Part print with two shaded views. Sizes in mm from the minimum x, y, z corner. A direction names the side the tool comes from. Round coordinates to 2 decimals unless told otherwise and drop trailing zeros. Order: outer loops, then holes, each group sorted by start corner. A loop starts at its lowest first (then second) coordinate and runs counter-clockwise, first axis right, second up. Notation, with made-up numbers: M 37.25,-13 L 77.25,-13 A8 cw 77.25,-7 Z; hole C 89,89.5 d9. An arc over 180 degrees is marked long. Answer as a JSON object with one key per item and string values.
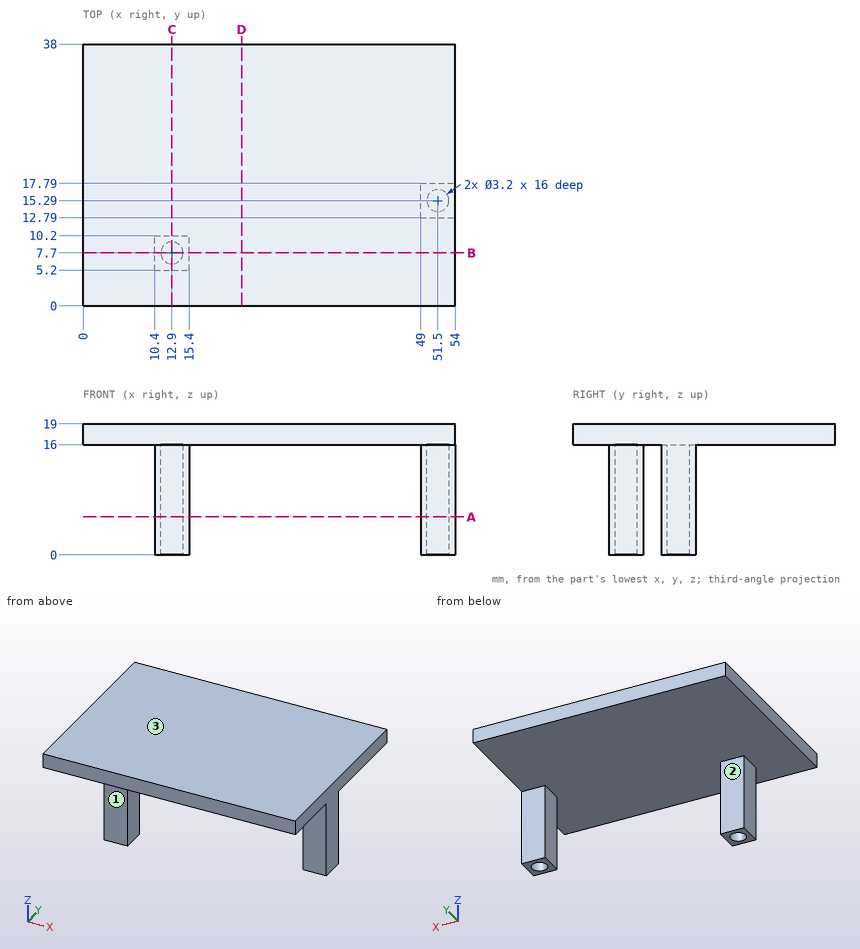
Item 1: Saw through at A-A on z = 5.5. List the corners of the cut face in (x, y).
Worked answers:
{"outline": "M 10.4,5.2 L 15.4,5.2 L 15.4,10.2 L 10.4,10.2 Z; M 49,12.79 L 54,12.79 L 54,17.79 L 49,17.79 Z; hole C 12.9,7.7 d3.2; hole C 51.5,15.29 d3.2"}
Item 2: 3-axis set-ups, long thin cutter, end or side, ignore diameter. For the marked faces 1, 2 and 3: which of +Z, -Z, +X, -X, +Y, -Y reach the whole face in a straight line?
Worked answers:
{"face 1": "-Z, +X, -X, -Y", "face 2": "-Z, +X, -X, +Y", "face 3": "+Z, +X, -X, +Y, -Y"}
Item 3: Saw through at C-C on x = 12.9. List the corners of the cut face in (y, z), and give its area (3 significant figures).
Worked answers:
{"outline": "M 0,16 L 5.2,16 L 5.2,0 L 6.1,0 L 6.1,16 L 9.3,16 L 9.3,0 L 10.2,0 L 10.2,16 L 38,16 L 38,19 L 0,19 Z", "area": "143 mm2"}
Item 4: Wall check: line 1 along Y through (x, z) = (51.5, 5.5); line 2 along Z through (x, y) = (46.5, 11); line 3 along X through (y, z) = (7.5, 14.25). Give the ranges that are in metal, low to high. Write a range as [from, to].
Worked answers:
{"line 1": "y = [12.79, 13.69], [16.89, 17.79]", "line 2": "z = [16, 19]", "line 3": "x = [10.4, 11.31], [14.49, 15.4]"}
Item 5: Saw through at D-D on x = 23. List the corners of the cut face in (y, z).
Worked answers:
{"outline": "M 0,16 L 38,16 L 38,19 L 0,19 Z"}
Item 6: Saw through at B-B on y = 7.7. List the corners of the cut face in (x, z), and give its area (3 significant figures).
Worked answers:
{"outline": "M 0,16 L 10.4,16 L 10.4,0 L 11.3,0 L 11.3,16 L 14.5,16 L 14.5,0 L 15.4,0 L 15.4,16 L 54,16 L 54,19 L 0,19 Z", "area": "191 mm2"}
Item 7: Drop flat-ended pins along their axis: pin 1 Ø2.5 at (x, z) = (52.5, 6.5) entering from -Y; pin 2 Ø5 at (x, z) = (41.5, 11.5) entering from -Y; pin 3 Ø4 at (y, z) = (8, 6.5) entering from +X; pin 4 Ø1.6 at (x, y) = (52, 15.5) entering from -Z. Give the stop position or say it passes through.
Worked answers:
{"pin 1": "stops at y = 12.79", "pin 2": "passes through", "pin 3": "stops at x = 15.4", "pin 4": "stops at z = 16"}
